from build123d import *

# Parameters (mm, degrees)
BOSS_EXTRUDE1_DEPTH = 10
BOSS_EXTRUDE2_DEPTH = 12
SKETCH7_R           = 1.95
CUT_EXTRUDE3_DEPTH  = 4
SKETCH8_R           = 1.95
CUT_EXTRUDE4_DEPTH  = 4
SKETCH9_R           = 1.5
CUT_EXTRUDE5_DEPTH  = 4
LPATTERN1_COUNT     = 2
LPATTERN1_PITCH     = 75
CHAMFER1_SIZE       = 9
LPATTERN2_COUNT     = 3
LPATTERN2_PITCH     = 75
SKETCH12_R          = 2.05
CUT_EXTRUDE6_DEPTH  = 4
SKETCH13_R          = 1.6
CUT_EXTRUDE8_DEPTH  = 5


with BuildPart() as part:
    # Sketch1 → Boss-Extrude1 (new body)
    with BuildSketch(Plane(origin=(0, 0, 0), x_dir=(1, 0, 0), z_dir=(0, 1, 0))):
        with BuildLine():
            Line((0, -11.5), (0, -31.5))
            Line((0, -31.5), (35, -31.5))
            Line((35, -31.5), (35, 181.5))
            Line((35, 181.5), (0, 181.5))
            Line((0, 181.5), (0, 161.5))
            ThreePointArc((0, 161.5), (11.5, 150), (0, 138.5))
            Line((0, 138.5), (0, 86.5))
            ThreePointArc((0, 86.5), (11.5, 75), (0, 63.5))
            Line((0, 63.5), (0, 11.5))
            ThreePointArc((0, 11.5), (11.5, 0), (0, -11.5))
        make_face()
    extrude(amount=-BOSS_EXTRUDE1_DEPTH)

    # Sketch3 → Boss-Extrude2 (add)
    with BuildSketch(Plane.XZ.offset(10)):
        with BuildLine():
            Line((0, -181.5), (0, -161.5))
            ThreePointArc((0, -161.5), (11.5, -150), (0, -138.5))
            Line((0, -138.5), (0, -86.5))
            ThreePointArc((0, -86.5), (11.5, -75), (0, -63.5))
            Line((0, -63.5), (0, -11.5))
            ThreePointArc((0, -11.5), (11.5, 0), (0, 11.5))
            Line((0, 11.5), (0, 31.5))
            Line((0, 31.5), (5, 31.5))
            Line((5, 31.5), (5, 15.724185194))
            ThreePointArc((5, 15.724185194), (16.5, 0), (5, -15.724185194))
            Line((5, -15.724185194), (5, -59.275814806))
            ThreePointArc((5, -59.275814806), (16.5, -75), (5, -90.724185194))
            Line((5, -90.724185194), (5, -134.275814806))
            ThreePointArc((5, -134.275814806), (16.5, -150), (5, -165.724185194))
            Line((5, -165.724185194), (5, -181.5))
            Line((5, -181.5), (0, -181.5))
        make_face()
    extrude(amount=BOSS_EXTRUDE2_DEPTH)

    # Sketch7 → Cut-Extrude3 (cut)
    with BuildSketch(Plane.ZY):
        with Locations((-170.5, -4)):
            Circle(SKETCH7_R)
        with Locations(Location((-170.5, -18, 0), (0, 0, 180))):
            Circle(SKETCH7_R)
        with Locations(Location((-129.5, -4, 0), (0, 0, 180))):
            Circle(SKETCH7_R)
        with Locations((-129.5, -18)):
            Circle(SKETCH7_R)
        with Locations((-95.5, -4)):
            Circle(SKETCH7_R)
        with Locations(Location((-54.5, -4, 0), (0, 0, 180))):
            Circle(SKETCH7_R)
        with Locations((-54.5, -18)):
            Circle(SKETCH7_R)
        with Locations(Location((-95.5, -18, 0), (0, 0, 180))):
            Circle(SKETCH7_R)
        with Locations((-20.5, -4)):
            Circle(SKETCH7_R)
        with Locations(Location((20.5, -4, 0), (0, 0, 180))):
            Circle(SKETCH7_R)
        with Locations((20.5, -18)):
            Circle(SKETCH7_R)
        with Locations(Location((-20.5, -18, 0), (0, 0, 180))):
            Circle(SKETCH7_R)
    extrude(amount=-CUT_EXTRUDE3_DEPTH, mode=Mode.SUBTRACT)

    # Sketch8 → Cut-Extrude4 (cut)
    with BuildSketch(Plane.ZY):
        with Locations((-112.5, -18.5)):
            Circle(SKETCH8_R)
    cut_extrude4 = extrude(amount=-CUT_EXTRUDE4_DEPTH, mode=Mode.SUBTRACT)

    # Sketch9 → Cut-Extrude5 (cut)
    with BuildSketch(Plane.ZY.offset(-4)):
        with Locations((-112.5, -18.5)):
            Circle(SKETCH9_R)
    cut_extrude5 = extrude(amount=-CUT_EXTRUDE5_DEPTH, mode=Mode.SUBTRACT)

    # LPattern1: Cut-Extrude4, Cut-Extrude5 ×2
    with Locations(*[(0, 0, i * LPATTERN1_PITCH) for i in range(1, LPATTERN1_COUNT)]):
        add(cut_extrude4, mode=Mode.SUBTRACT)
        add(cut_extrude5, mode=Mode.SUBTRACT)

    # Chamfer1
    chamfer1_edges = [part.edges().sort_by_distance(p)[0] for p in [
        (35, -10, -75),
    ]]
    chamfer(chamfer1_edges, length=CHAMFER1_SIZE)

    # Sketch10 → Cut-Revolve1 (revolve, cut)
    with BuildSketch(Plane.ZY):
        with BuildLine():
            Line((-161.5, 0), (-161.5, -6.48))
            ThreePointArc((-161.5, -6.48), (-162.959732838, -5.143785702), (-163.5, -3.24))
            Line((-163.5, -3.24), (-163.5, 0))
            Line((-163.5, 0), (-161.5, 0))
        make_face()
    cut_revolve1 = revolve(axis=Axis((0, 19.009810116, -150), (0, -1, 0)), mode=Mode.SUBTRACT)

    # LPattern2: Cut-Revolve1 ×3
    with Locations(*[(0, 0, i * LPATTERN2_PITCH) for i in range(1, LPATTERN2_COUNT)]):
        add(cut_revolve1, mode=Mode.SUBTRACT)

    # Sketch12 → Cut-Extrude6 (cut)
    with BuildSketch(Plane(origin=(0, 0, 0), x_dir=(1, 0, 0), z_dir=(0, 1, 0))):
        with Locations(Location((20, -21.5, 0), (0, 0, 270))):
            Circle(SKETCH12_R)
    cut_extrude6 = extrude(amount=-CUT_EXTRUDE6_DEPTH, mode=Mode.SUBTRACT)

    # Sketch13 → Cut-Extrude8 (cut)
    with BuildSketch(Plane(origin=(0, -4, 0), x_dir=(1, 0, 0), z_dir=(0, 1, 0))):
        with Locations(Location((20, -21.5, 0), (0, 0, 270))):
            Circle(SKETCH13_R)
    cut_extrude8 = extrude(amount=-CUT_EXTRUDE8_DEPTH, mode=Mode.SUBTRACT)

    # Mirror2: Cut-Extrude6, Cut-Extrude8 across plane
    add(cut_extrude6.mirror(Plane.XY.offset(-75)), mode=Mode.SUBTRACT)
    add(cut_extrude8.mirror(Plane.XY.offset(-75)), mode=Mode.SUBTRACT)


solid = part.part
Check sheet for the modelled part. Datum: model origin and axes. Units: mm. A direction names the side the tool comes from. Give positions to 0.01 mm unless a question says otherwise; leave off trailing zeros. Loops run counter-clockwise (first coordinate to the right, second up) from the corner with the lowest first, then second, coordinate; pieces in that order, holes last. Notation, with made-up numbers: M 34.5,-5 L 91.5,-5 A25 cw 91.5,27 Z; hole C -35,-12.75 d8. An arc over 180 degrees is marked long. Use a Markdown table: item, result. Add a question column.
Q1. Sectioned sample at C-C, the plane x = 31.5. Record the cut outline in (y, z).
Q2. Sectioned sample at B-B, the plane y = -13.25. Record the cut outline in (x, z).
Q3. Mould release check, pull along Z, two halves, no side actions. Record for faces 4 (the flat face through (17, 0, -76)), 5 (the cylindrical face through (1.972, -16.813, -93.953)), 6 (the flat face through (4, -18, -130)), 7 (the flat face through (14, -6, -181.5)): pulls with the +Z half, pulls with the -Z half, needs draft (parallel to the pull), parting line crosses it, or undercut.
Q4. Tool access check on faces 1 (the flat face through (5, -16, -174)), 2 (the cylindrical face through (1.97, -3.25, -56.3)), 3 (the cylindrical face through (16.497, -15.916, -74.708)). Record the directions out of +Z, -Z, +X, -X, +Y, -Y that give a thin tool (end or side, any length) a straight path to the whole face; none if there is none.
Q5. Scan lines: line 1 along Y through (x, z) = (1.4, -54.5); line 2 along Z through (x, y) = (13, -18); line 3 along Y through (x, z) = (21, -86). Record each from-to range of solid material in increasing order. Write a range as [from, to].
Q6. Go/stop test with flat-tipped pins: pin 1 (1.2 mm diameter, centred on y = -18, z = -112, fed in from -X); pin 2 (1.9 mm diameter, centred on x = 20, z = -171.5, fed in from -Y); pin 3 (9.5 mm diameter, centred on y = -13.5, z = -175, fed in from +X); pin 4 (6 mm diameter, centred on y = -11.5, z = -59.5, fed in from +X). Record where each tip stops, or that it passes through.
Q7. Sectioned sample at A-A, the plane z = -150. Record the cut outline in (x, y), then the cut area to 3 significant figures.
Q8. Sectioned sample at D-D, the plane z = -43. Record the cut outline in (x, y), then the cut area to 4 significant figures.
Verdict:
| question | item | result |
|---|---|---|
| 1 | outline | M -4.5,-181.5 L 0,-181.5 L 0,31.5 L -4.5,31.5 Z |
| 2 | outline | M 0,-181.5 L 5,-181.5 L 5,-165.72 A16.5 ccw 5,-134.28 L 5,-90.72 A16.5 ccw 5,-59.28 L 5,-15.72 A16.5 ccw 5,15.72 L 5,31.5 L 0,31.5 L 0,11.5 A11.5 cw 0,-11.5 L 0,-63.5 A11.5 cw 0,-86.5 L 0,-138.5 A11.5 cw 0,-161.5 Z |
| 3 | face 4 | needs draft |
| 3 | face 5 | undercut |
| 3 | face 6 | undercut |
| 3 | face 7 | pulls with the -Z half |
| 4 | face 1 | -Z, +X, -Y |
| 4 | face 2 | -X |
| 4 | face 3 | +X, -Y |
| 5 | line 1 | [-22, -19.95], [-16.05, -5.95], [-2.05, 0] |
| 5 | line 2 | [-160.16, -139.84], [-85.16, -64.84], [-10.16, 10.16] |
| 5 | line 3 | [-10, 0] |
| 6 | pin 1 | through |
| 6 | pin 2 | y = -10 |
| 6 | pin 3 | x = 27.25 |
| 6 | pin 4 | x = 27.5 |
| 7 | outline | M 11.5,-22 L 16.5,-22 L 16.5,-10 L 26,-10 L 35,-1 L 35,0 L 13.5,0 L 13.5,-3.24 A3.62 cw 11.5,-6.48 Z |
| 7 | area | 243 mm^2 |
| 8 | outline | M 0,-22 L 5,-22 L 5,-10 L 26,-10 L 35,-1 L 35,0 L 0,0 Z |
| 8 | area | 369.5 mm^2 |
